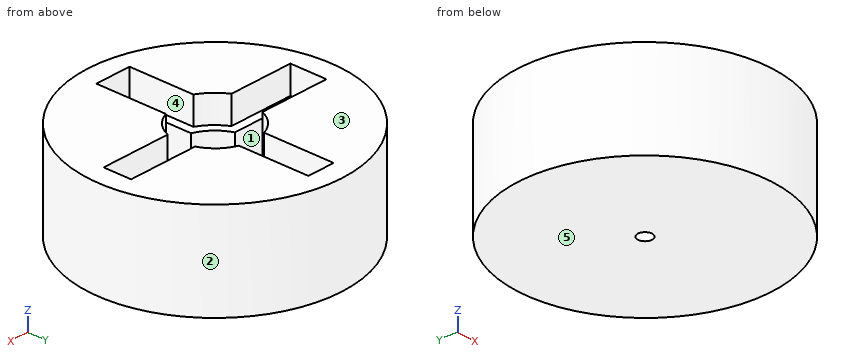
```python
from build123d import *

# Parameters (mm, degrees)
F3_DEPTH = 13.4
F5_R     = 2.89999
F6_R     = 0.5
F7_DEPTH = 5.7


# Not quite as in the source:
# - a fillet or chamfer is up to 0.001 mm smaller than in the source, because OpenCascade refuses the exact size


with BuildPart() as f1:
    # F0 (on Right) → F1 (revolve)
    with BuildSketch(Plane.YZ):
        Polygon((1.5, 10.2), (1.5, 0), (26.75, 0), (26.75, 20), (4.125, 20), (4.125, 10.2), align=None)
    revolve(axis=Axis((0, 0, 0.3519081866), (0, 0, -1)))

    # F2 (on face) → F3 (cut)
    with BuildSketch(Plane.XY.offset(20)):
        with BuildLine():
            Line((-22.4, 2.9), (-22.4, -2.9))
            Line((-22.4, -2.9), (-7.7235030912, -2.9))
            ThreePointArc((-7.7235030912, -2.9), (-8.25, 0), (-7.7235030912, 2.9))
            Line((-7.7235030912, 2.9), (-22.4, 2.9))
        make_face()
        with BuildLine():
            ThreePointArc((-7.7235030912, 2.9), (-8.25, 0), (-7.7235030912, -2.9))
            Line((-7.7235030912, -2.9), (-2.9, -2.9))
            Line((-2.9, -2.9), (-2.9, 2.9))
            Line((-2.9, 2.9), (-7.7235030912, 2.9))
        make_face()
        with BuildLine():
            Line((-2.9, -2.9), (-7.7235030912, -2.9))
            ThreePointArc((-7.7235030912, -2.9), (-5.8336309448, -5.8336309448), (-2.9, -7.7235030912))
            Line((-2.9, -7.7235030912), (-2.9, -2.9))
        make_face()
        with BuildLine():
            Line((2.9, -2.9), (-2.9, -2.9))
            Line((-2.9, -2.9), (-2.9, -7.7235030912))
            ThreePointArc((-2.9, -7.7235030912), (0, -8.25), (2.9, -7.7235030912))
            Line((2.9, -7.7235030912), (2.9, -2.9))
        make_face()
        with BuildLine():
            ThreePointArc((-2.9, 7.7235030912), (-5.8336309448, 5.8336309448), (-7.7235030912, 2.9))
            Line((-7.7235030912, 2.9), (-2.9, 2.9))
            Line((-2.9, 2.9), (-2.9, 7.7235030912))
        make_face()
        with BuildLine():
            ThreePointArc((2.9, -7.7235030912), (0, -8.25), (-2.9, -7.7235030912))
            Line((-2.9, -7.7235030912), (-2.9, -22.4))
            Line((-2.9, -22.4), (2.9, -22.4))
            Line((2.9, -22.4), (2.9, -7.7235030912))
        make_face()
        with BuildLine():
            Line((2.9, 2.9), (2.9, -2.9))
            Line((2.9, -2.9), (7.7235030912, -2.9))
            ThreePointArc((7.7235030912, -2.9), (8.1173086828, -1.4737027342), (8.25, 0))
            ThreePointArc((8.25, 0), (8.1173086828, 1.4737027342), (7.7235030912, 2.9))
            Line((7.7235030912, 2.9), (2.9, 2.9))
        make_face()
        with BuildLine():
            Line((7.7235030912, -2.9), (2.9, -2.9))
            Line((2.9, -2.9), (2.9, -7.7235030912))
            ThreePointArc((2.9, -7.7235030912), (5.8336309448, -5.8336309448), (7.7235030912, -2.9))
        make_face()
        with BuildLine():
            Line((-2.9, 7.7235030912), (-2.9, 2.9))
            Line((-2.9, 2.9), (2.9, 2.9))
            Line((2.9, 2.9), (2.9, 7.7235030912))
            ThreePointArc((2.9, 7.7235030912), (0, 8.25), (-2.9, 7.7235030912))
        make_face()
        with BuildLine():
            Line((-2.9, 22.4), (-2.9, 7.7235030912))
            ThreePointArc((-2.9, 7.7235030912), (0, 8.25), (2.9, 7.7235030912))
            Line((2.9, 7.7235030912), (2.9, 22.4))
            Line((2.9, 22.4), (-2.9, 22.4))
        make_face()
        with BuildLine():
            ThreePointArc((8.25, 0), (8.1173086828, -1.4737027342), (7.7235030912, -2.9))
            Line((7.7235030912, -2.9), (22.4, -2.9))
            Line((22.4, -2.9), (22.4, 2.9))
            Line((22.4, 2.9), (7.7235030912, 2.9))
            ThreePointArc((7.7235030912, 2.9), (8.1173086828, 1.4737027342), (8.25, 0))
        make_face()
        with BuildLine():
            Line((2.9, 7.7235030912), (2.9, 2.9))
            Line((2.9, 2.9), (7.7235030912, 2.9))
            ThreePointArc((7.7235030912, 2.9), (5.8336309448, 5.8336309448), (2.9, 7.7235030912))
        make_face()
    extrude(amount=-F3_DEPTH, mode=Mode.SUBTRACT)

    # F5 (radius 2.9 in the source; OpenCascade refuses exactly that, so slightly less here)
    f5_edges = [f1.edges().sort_by_distance(p)[0] for p in [
        (2.9, 2.9, 8.4),
        (-2.9, -2.9, 8.4),
        (-2.9, 2.9, 8.4),
        (2.9, -2.9, 8.4),
    ]]
    fillet(f5_edges, radius=F5_R)

    # F6
    f6_edges = [f1.edges().sort_by_distance(p)[0] for p in [
        (-2.050613, -2.050613, 6.6),
        (-2.050613, -2.050613, 10.2),
    ]]
    fillet(f6_edges, radius=F6_R)

    # F4 (on face) → F7 (cut)
    with BuildSketch(Plane.XY.offset(20)):
        with BuildLine():
            Line((-4.7, -8.883270794), (-4.7, -22.4))
            Line((-4.7, -22.4), (-2.9, -22.4))
            Line((-2.9, -22.4), (-2.9, -7.7235030912))
            ThreePointArc((-2.9, -7.7235030912), (-5.8336309448, -5.8336309448), (-7.7235030912, -2.9))
            Line((-7.7235030912, -2.9), (-22.4, -2.9))
            Line((-22.4, -2.9), (-22.4, -4.7))
            Line((-22.4, -4.7), (-8.883270794, -4.7))
            ThreePointArc((-8.883270794, -4.7), (-7.1064231509, -7.1064231509), (-4.7, -8.883270794))
        make_face()
    extrude(amount=-F7_DEPTH, mode=Mode.SUBTRACT)


solid = f1.part
```
The model under review builds one solid part; all positions refer to its coordinate system, in mm. Face numbers are marked on the shaded views. A direction names the side the tool comes from. Round coordinates to 2 decimals unless told otherwise and drop trailing zeros. Write each loop counter-clockwise with the first axis right and the second up, starting at its lowest first coordinate (ties: lowest second). Pieces come first, ordered by that corner, then holes.
(1) We need section D-D on x = 9. Give the boundary of the cut face in (y, z).
(2) We need section A-A on z = 7.75. Give the number of separate pieces and of enclosed holes in the cut face, and give its area (3 significant figures).
(3) Insertion check: pin 1 (12 mm diameter, centred on y = 3, z = 15, fed in from -X); pin 2 (10.5 mm diameter, centred on x = 16.5, z = 10.5, fed in from +Y); pin 3 (2 mm diameter, centred on y = 17.5, z = 3.5, fed in from +X) (3 decimals). Each pin has a flat end and moves straight along its axis. Give the tip position at first contact, or say it passes through.
(4) Machinability: for the marked faces 4 and 5, which of the approach directions +Z, -Z, +X, -X, +Y, -Y give a long, thin tool a straight path to every point of the face, cutting with its end or side? Answer none if there is none.
(5) Mouldability with a two-part tool opening along Y and no side actions: class the marked faces 1, 2 and 3 as +Y half, -Y half, draft (parallel to the pull), parting line (faces both ways), or undercut.
(6) Wall thickness on L1, parallel to X at y = 0, z = 7.75; L2, parallel to X at y = 0, z = 3.5; L3, parallel to Z at x = -9.5, y = 2: over which ranges is each line inside the solid? List them lowest first.
(7) We need section C-C on y = 14.5. Give the boundary of the cut face in (x, z).
(8) We need section B-B on z = 13.5. Give the boundary of the cut face in (x, y).
Findings below:
1. outline: (-25.19, 0) - (25.19, 0) - (25.19, 20) - (2.9, 20) - (2.9, 6.6) - (-2.9, 6.6) - (-2.9, 20) - (-25.19, 20) - close
2. separate pieces: 2
2. enclosed holes: 2
2. area: 1,720 mm2
3. pin 1: stops at x = -26.75
3. pin 2: stops at y = 24.27
3. pin 3: stops at x = 21.055
4. face 4: +Z
4. face 5: -Z, +X, -X, +Y, -Y
5. face 1: undercut
5. face 2: parting line
5. face 3: draft
6. L1: x = -26.75 to -22.4, -2.9 to -1.5, 1.5 to 2.9, 22.4 to 26.75
6. L2: x = -26.75 to -1.5, 1.5 to 26.75
6. L3: z = 0 to 6.6
7. outline: (-22.48, 0) - (22.48, 0) - (22.48, 20) - (2.9, 20) - (2.9, 6.6) - (-2.9, 6.6) - (-2.9, 20) - (-22.48, 20) - close
8. outline: circle Ø53.5 at (0, 0); hole (-22.4, -2.9) - (-7.72, -2.9) arc R8.25 ccw to (-2.9, -7.72) - (-2.9, -22.4) - (2.9, -22.4) - (2.9, -7.72) arc R8.25 ccw to (7.72, -2.9) - (22.4, -2.9) - (22.4, 2.9) - (7.72, 2.9) arc R8.25 ccw to (2.9, 7.72) - (2.9, 22.4) - (-2.9, 22.4) - (-2.9, 7.72) arc R8.25 ccw to (-7.72, 2.9) - (-22.4, 2.9) - close
